Part model, mm, in its own coordinate system. A direction names the side the tool comes from. Give positions to 0.01 mm unless a question says otherwise; leave off trailing zeros. Order: outer loops, then holes, each group sorted by start corner. A loop starts at its lowest first (then second) coordinate and runs counter-clockwise, first axis right, second up. Notation, with made-up numbers: (85.25, 53.25) - (105.25, 53.25) arc R15 ccw to (105.25, 66.25) - close; hole circle Ø10 at (47, 50.5). An arc over 180 degrees is marked (long way). One line per item, written item: value.
```python
from build123d import *

# Parameters (mm, degrees)
BOSS_EXTRU_1_DEPTH = 65
CHANFREIN4_SIZE    = 20
CHANFREIN5_SIZE    = 20


with BuildPart() as part:
    # Esquisse1 → Boss.-Extru.1 (new body)
    with BuildSketch(Plane(origin=(0, 0, 0), x_dir=(0, 0, -1), z_dir=(1, 0, 0))):
        Polygon((-20.69418762, -12.633516796), (19.30581238, -12.633516796), (19.30581238, 17.366483204), (9.30581238, 17.366483204), (9.30581238, 32.366483204), (-5.69418762, 32.366483204), (-5.69418762, 2.366483204), (-20.69418762, 2.366483204), align=None)
    extrude(amount=BOSS_EXTRU_1_DEPTH)

    # Chanfrein4
    chanfrein4_edges = [part.edges().sort_by_distance(p)[0] for p in [
        (65, 32.366483204, -1.80581238),
    ]]
    chamfer(chanfrein4_edges, length=CHANFREIN4_SIZE)

    # Chanfrein5
    chanfrein5_edges = [part.edges().sort_by_distance(p)[0] for p in [
        (0, 32.366483204, -1.80581238),
    ]]
    chamfer(chanfrein5_edges, length=CHANFREIN5_SIZE)


solid = part.part
```
1) Wall check: line 1 along Z through (x, y) = (49.5, 13.5); line 2 along Z through (x, y) = (16, 22.5); line 3 along Y through (x, z) = (40.5, -15). Give the ranges that are in metal, low to high. Write a range as [from, to].
Answer:
line 1: z = [-19.31, 5.69]
line 2: z = [-9.31, 5.69]
line 3: y = [-12.63, 17.37]
2) Slice it at B-B on x = 27.5. Write the cut outline in (y, z), then the cut area to 3 significant figures.
Answer:
outline: (-12.63, -19.31) - (17.37, -19.31) - (17.37, -9.31) - (32.37, -9.31) - (32.37, 5.69) - (2.37, 5.69) - (2.37, 20.69) - (-12.63, 20.69) - close
area: 1,200 mm2
3) Slice it at C-C on y = 6.5. Write the cut outline in (x, z).
Answer:
outline: (0, -19.31) - (65, -19.31) - (65, 5.69) - (0, 5.69) - close
4) Slice it at D-D on z = -12. Write the cut outline in (x, y), then the cut area to 4 significant figures.
Answer:
outline: (0, -12.63) - (65, -12.63) - (65, 12.37) - (60, 17.37) - (5, 17.37) - (0, 12.37) - close
area: 1,925 mm2
5) Which spindle directions (+Z, -Z, +X, -X, +Y, -Y) get a long thin tool onto all of the face, cutting with end or side? Do faces 1 (the face through (65, 0, -3)), 2 (the face through (32, 17.366, -14)), 3 (the face through (32, 2.366, 13)). Say none if no direction does.
Answer:
face 1: +Z, -Z, +X, +Y, -Y
face 2: -Z, +X, -X, +Y
face 3: +Z, +X, -X, +Y
6) Drop flat-ended pins along their axis: P1, Ø5, axis at x = 26, z = -12.5, coming from the +Y side; P2, Ø12, axis at x = 36, z = 13, coming from the +Y side; P3, Ø3, axis at x = 39.5, y = 20.5, coming from the +Z side. Give the stop position or say it passes through.
Answer:
P1: stops at y = 17.37
P2: stops at y = 2.37
P3: stops at z = 5.69
7) Slice it at A-A on z = -1. Write the cut outline in (x, y).
Answer:
outline: (0, -12.63) - (65, -12.63) - (65, 12.37) - (45, 32.37) - (20, 32.37) - (0, 12.37) - close
